from build123d import *

# Parameters (mm, degrees)
BOSS_EXTRUDE1_START = -39.622072
BOSS_EXTRUDE1_DEPTH = 95.622072
SKETCH3_OUTSIDE_W   = 79.464
SKETCH3_OUTSIDE_H   = 119.774
CUT_EXTRUDE1_DEPTH  = 63.967259819


with BuildPart() as part:
    # Sketch2 → Boss-Extrude1 (new body)
    with BuildSketch(Plane.XY.offset(BOSS_EXTRUDE1_START)):
        Polygon((23.948813845, 0), (27.656388216, -7.053975388), (27.005057694, -8), (-27.005057694, -8), (-27.656388216, -7.053975388), (-23.948813845, 0), align=None)
    extrude(amount=BOSS_EXTRUDE1_DEPTH)

    # Sketch3 outside → Cut-Extrude1 (cut, through all)
    with BuildSketch(Plane(origin=(0, 0, 0), x_dir=(1, 0, 0), z_dir=(0, 1, 0))):
        with Locations((0, -8.189)):
            Rectangle(SKETCH3_OUTSIDE_W, SKETCH3_OUTSIDE_H)
        Polygon((0, 32.635105346), (8.326742195, 39.622071651), (27.656388216, 20.292425629), (27.656388216, -51.380750229), (0, -56), (-27.656388216, -51.380750229), (-27.656388216, 20.292425629), (-8.326742195, 39.622071651), align=None, mode=Mode.SUBTRACT)
    extrude(amount=-CUT_EXTRUDE1_DEPTH, mode=Mode.SUBTRACT)


solid = part.part
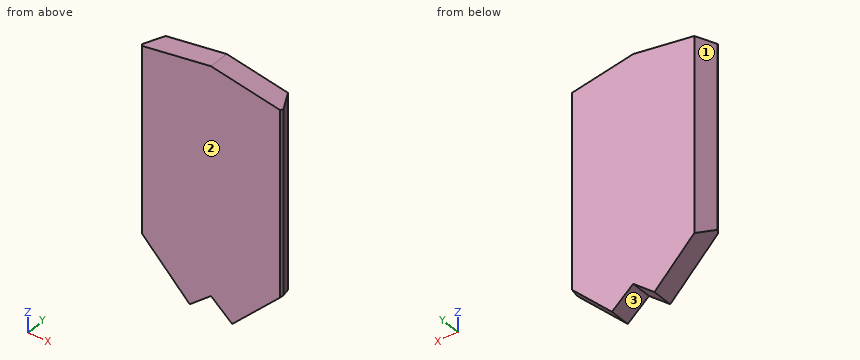
Design review of the part built by this model. Coordinates are the model's own, in mm. Face numbers are marked on the shaded views. Round coordinates to 2 decimals unless told otherwise and drop trailing zeros. Write each loop counter-clockwise with the first axis right and the second up, starting at its lowest first coordinate (ties: lowest second). Pieces come first, ordered by that corner, then holes. Notation, with made-up numbers: (69, 25.25) - (93, 25.25) arc R22 cw to (93, 46.25) - close; hole circle Ø4 at (61.5, 0). An arc over 180 degrees is marked (long way). Use a Markdown table: item, result. Add a question column.
1. We need section D-D (y = -6). State the section outline as (x, z) points, then the cut area to 3 significant figures.
2. Clearance check with flat-ended pins moving along their axes: pin 1 (4 mm diameter, centred on y = -3, z = 9.5, fed in from +X); pin 2 (4 mm diameter, centred on x = 14.5, y = -5, fed in from -Z); pin 3 (1 mm diameter, centred on y = -6.5, z = 40, fed in from -X). State where each tip first meets the part, or that it passes through.
3. Wall thickness on probe 1 along Z at (x, y) = (-24, -4.25); probe 2 along X at (y, z) = (-0.5, -24); probe 3 along X at (y, z) = (-2.75, -20.5): over which ranges is each line inside the solid? List them lowest first.
4. We need section A-A (z = 1.5). State the section outline as (x, y) points, then the cut area to 3 significant figures.
5. We need section C-C (x = 4.5). State the section outline as (y, z) points, then the cut area to 3 significant figures.
6. Mouldability with a two-part tool opening along X and no side actions: class the marked faces 1, 2 and 3 as +X half, -X half, draft (parallel to the pull), parting line (faces both ways), or undercut.
7. We need section B-B (y = -1). State the section outline as (x, z) points.
Output:
| question | item | result |
|---|---|---|
| 1 | outline | (-27.1, -20.85) - (-8.33, -39.62) - (0, -32.64) - (8.33, -39.62) - (27.1, -20.85) - (27.1, 51.47) - (0, 56) - (-27.1, 51.47) - close |
| 1 | area | 4,650 mm2 |
| 2 | pin 1 | stops at x = 26.58 |
| 2 | pin 2 | stops at z = -35.45 |
| 2 | pin 3 | stops at x = -27.63 |
| 3 | probe 1 | z = -23.95 to 51.99 |
| 3 | probe 2 | x = -23.95 to 23.95 |
| 3 | probe 3 | x = -25.39 to 25.39 |
| 4 | outline | (-27.66, -7.05) - (-27.01, -8) - (27.01, -8) - (27.66, -7.05) - (23.95, 0) - (-23.95, 0) - close |
| 4 | area | 416 mm2 |
| 5 | outline | (-8, -36.41) - (0, -36.41) - (0, 55.25) - (-8, 55.25) - close |
| 5 | area | 733 mm2 |
| 6 | face 1 | -X half |
| 6 | face 2 | draft |
| 6 | face 3 | undercut |
| 7 | outline | (-24.47, -23.47) - (-8.33, -39.62) - (0, -32.64) - (8.33, -39.62) - (24.47, -23.47) - (24.47, 51.91) - (0, 56) - (-24.47, 51.91) - close |
